```python
from build123d import *

# Parameters (mm, degrees)
BOSS_EXTRUDE1_START     = -3
BOSS_EXTRUDE1_OUTLINE_R = 1.5
BOSS_EXTRUDE1_DEPTH     = 3
FILLET1_R               = 0.5


# Read off the part's stored shape, not the designer's step: Boss-Extrude1
with BuildPart() as part:
    # Boss-Extrude1 outline → Boss-Extrude1 (new body)
    with BuildSketch(Plane.XY.offset(BOSS_EXTRUDE1_START)):
        with BuildLine():
            Line((11.834428484, -2.472731782), (31.256409707, 0.084220555))
            ThreePointArc((31.256409707, 0.084220555), (34.700084383, 4.572104769), (30.212200169, 8.015779445))
            Line((30.212200169, 8.015779445), (13.428337838, 5.806142051))
            ThreePointArc((13.428337838, 5.806142051), (13.411032377, 5.846003182), (13.39360859, 5.885812734))
            ThreePointArc((13.39360859, 5.885812734), (12.04167814, 5.897146383), (10.729304164, 5.572309592))
            Line((10.729304164, 5.572309592), (10.189200244, 6.507557022))
            ThreePointArc((10.189200244, 6.507557022), (11.126720661, 7.481723913), (11.792869471, 8.658240563))
            ThreePointArc((11.792869471, 8.658240563), (11.606759368, 8.906179706), (11.415437385, 9.150119633))
            ThreePointArc((11.415437385, 9.150119633), (10.106597569, 8.81117421), (8.922976471, 8.15773197))
            ThreePointArc((8.922976471, 8.15773197), (8.549706323, 8.548135574), (8.159371308, 8.921477448))
            ThreePointArc((8.159371308, 8.921477448), (8.812813548, 10.105098546), (9.151758972, 11.413938362))
            Line((9.151758972, 11.413938362), (8.659879901, 11.791370448))
            ThreePointArc((8.659879901, 11.791370448), (7.483516811, 11.125336137), (6.509436976, 10.187999326))
            ThreePointArc((6.509436976, 10.187999326), (6.047829045, 10.468613272), (5.574146563, 10.728326528))
            ThreePointArc((5.574146563, 10.728326528), (5.898805358, 12.040487702), (5.887415057, 13.392168338))
            Line((5.887415057, 13.392168338), (5.314609747, 13.629432066))
            ThreePointArc((5.314609747, 13.629432066), (4.351003751, 12.681995862), (3.65280527, 11.524977816))
            ThreePointArc((3.65280527, 11.524977816), (3.134170467, 11.676689406), (2.609274564, 11.805074597))
            ThreePointArc((2.609274564, 11.805074597), (2.58305967, 13.15599481), (2.222297371, 14.458117388))
            Line((2.222297371, 14.458117388), (1.607601557, 14.539043627))
            ThreePointArc((1.607601557, 14.539043627), (0.922327421, 13.375148622), (0.547316802, 12.077605074))
            ThreePointArc((0.547316802, 12.077605074), (0.006856042, 12.089998056), (-0.533618427, 12.078218055))
            ThreePointArc((-0.533618427, 12.078218055), (-0.908651119, 13.375486662), (-1.593822374, 14.539142845))
            Line((-1.593822374, 14.539142845), (-2.208518188, 14.458216606))
            ThreePointArc((-2.208518188, 14.458216606), (-2.569071942, 13.157522433), (-2.595800172, 11.808044777))
            ThreePointArc((-2.595800172, 11.808044777), (-3.121351418, 11.680122659), (-3.640655008, 11.528821757))
            ThreePointArc((-3.640655008, 11.528821757), (-4.338480819, 12.683812024), (-5.300881923, 13.629722958))
            Line((-5.300881923, 13.629722958), (-5.873687233, 13.39245923))
            ThreePointArc((-5.873687233, 13.39245923), (-5.885433032, 12.043808909), (-5.562611018, 10.734312212))
            ThreePointArc((-5.562611018, 10.734312212), (-6.037455135, 10.474599539), (-6.500199913, 10.193895285))
            ThreePointArc((-6.500199913, 10.193895285), (-7.47268922, 11.127885908), (-8.646251294, 11.791833189))
            Line((-8.646251294, 11.791833189), (-9.138130365, 11.414401103))
            ThreePointArc((-9.138130365, 11.414401103), (-8.80083054, 10.109699304), (-8.150983569, 8.92914144))
            ThreePointArc((-8.150983569, 8.92914144), (-8.542690029, 8.555147402), (-8.917254459, 8.163986338))
            ThreePointArc((-8.917254459, 8.163986338), (-10.097571821, 8.813551755), (-11.401949093, 9.15072269))
            Line((-11.401949093, 9.15072269), (-11.779381179, 8.658843619))
            ThreePointArc((-11.779381179, 8.658843619), (-11.116550367, 7.486781519), (-10.184349411, 6.515145975))
            ThreePointArc((-10.184349411, 6.515145975), (-10.46607819, 6.052215075), (-10.726778871, 5.577124264))
            ThreePointArc((-10.726778871, 5.577124264), (-12.034053776, 5.89841947), (-13.38017907, 5.886378776))
            Line((-13.38017907, 5.886378776), (-13.617442798, 5.313573465))
            ThreePointArc((-13.617442798, 5.313573465), (-12.674640857, 4.353631081), (-11.523783462, 3.656571444))
            ThreePointArc((-11.523783462, 3.656571444), (-11.67614775, 3.13618777), (-11.805025713, 2.60949572))
            ThreePointArc((-11.805025713, 2.60949572), (-13.149945407, 2.581153618), (-14.44612812, 2.221261089))
            Line((-14.44612812, 2.221261089), (-14.527054359, 1.606565275))
            ThreePointArc((-14.527054359, 1.606565275), (-13.368714152, 0.923687604), (-12.07756623, 0.548173302))
            ThreePointArc((-12.07756623, 0.548173302), (-12.089998597, 0.005825389), (-12.07808888, -0.536534252))
            ThreePointArc((-12.07808888, -0.536534252), (-13.369010177, -0.912066026), (-14.527153576, -1.594858655))
            Line((-14.527153576, -1.594858655), (-14.446227337, -2.20955447))
            ThreePointArc((-14.446227337, -2.20955447), (-13.151251636, -2.569269431), (-11.807551859, -2.598041398))
            ThreePointArc((-11.807551859, -2.598041398), (0.064079741, -12.08983018), (11.834428484, -2.472731782))
        make_face()
        Circle(BOSS_EXTRUDE1_OUTLINE_R, mode=Mode.SUBTRACT)
        with Locations((30.734304938, 4.05)):
            Circle(BOSS_EXTRUDE1_OUTLINE_R, mode=Mode.SUBTRACT)
    extrude(amount=BOSS_EXTRUDE1_DEPTH)

    # Fillet1
    fillet1_edges = [part.edges().sort_by_distance(p)[0] for p in [
        (29.234304938, 4.05, -3),
        (29.234304938, 4.05, 0),
        (-1.5, 0, 0),
        (-1.5, 0, -3),
    ]]
    fillet(fillet1_edges, radius=FILLET1_R)


solid = part.part
```
Check sheet for the modelled part. Datum: model origin and axes. Units: mm. A direction names the side the tool comes from. Coordinates: 2 decimals unless noted, no trailing zeros. Write each loop counter-clockwise with the first axis right and the second up, starting at its lowest first coordinate (ties: lowest second). Pieces come first, ordered by that corner, then holes. Notation, with made-up numbers: (-10, 40.5) - (38, 40.5) arc R22 ccw to (38, 48.5) - close; hole circle Ø4 at (65.25, 68). An arc over 180 degrees is marked (long way). One line per question, with ' | ' between items.
Item 1: Sectioned sample at C-C on x = 24.5. Record the boundary of the cut face in (y, z).
Determined:
outline: (-0.81, -3) - (7.26, -3) - (7.26, 0) - (-0.81, 0) - close
Item 2: Mould release check, pull along X, two halves, no side actions. Record for faces 6 (the face through (21.409, -1.212, -1.521)), 7 (the face through (-10.08, 8.807, -1.521)), 8 (the face through (-13.386, 0.931, -1.521)): pulls with the +X half, pulls with the -X half, needs draft (parallel to the pull), parting line crosses it, or undercut.
Determined:
face 6: pulls with the +X half | face 7: undercut | face 8: pulls with the -X half
Item 3: Access from +Z, -Z, +X, -X, +Y, -Y to the whole of each face (thin tool, end or side, straight path). Record for faces 1 (the face through (-11.128, 7.502, -1.521)), 2 (the face through (4, 1, -3)), 3 (the face through (4, 1, 0)), 4 (the face through (10.463, 6.033, -1.521)), 5 (the face through (-0.9, 13.36, -1.52)).
Determined:
face 1: +Z, -Z, -X | face 2: -Z, +X, -X, +Y, -Y | face 3: +Z, +X, -X, +Y, -Y | face 4: +Z, -Z | face 5: +Z, -Z, +Y
Item 4: Thickness scan on line 1 (Y direction, x = 0, z = -1.95); line 2 (X direction, y = -4, z = -2.8); line 3 (Y direction, x = -12, z = -2). Record the ranges inside material, lowest first. Write a range as [from, to].
Determined:
line 1: y = [-12.09, -1.5], [1.5, 12.09] | line 2: x = [-11.41, 11.41] | line 3: y = [-2.61, 2.63], [3.9, 5.89]
Item 5: Sectioned sample at D-D on y = -8.25. Record the boundary of the cut face in (x, z), plus the area to 3 significant figures.
Determined:
outline: (-8.84, -3) - (8.84, -3) - (8.84, 0) - (-8.84, 0) - close | area: 53.0 mm2
Item 6: Gauge pin test, flat end, axial feed: P1, Ø3.5, axis at x = 30.73, y = 4.05, coming from the +Z side. Record the tip position at first contact, or that the pin passes through.
Determined:
P1: stops at z = -0.06
Item 7: Sectioned sample at A-A on x = 0. Record the boundary of the cut face in (y, z).
Determined:
outline: (-12.09, -3) - (-2, -3) arc R0.5 ccw to (-1.5, -2.5) - (-1.5, -0.5) arc R0.5 ccw to (-2, 0) - (-12.09, 0) - close; (1.5, -2.5) arc R0.5 ccw to (2, -3) - (12.09, -3) - (12.09, 0) - (2, 0) arc R0.5 ccw to (1.5, -0.5) - close
Item 8: Sectioned sample at B-B on z = -1.55. Give the number of separate pieces and of enclosed holes in the cut face, plus the area to 3 significant figures.
Determined:
separate pieces: 1 | enclosed holes: 2 | area: 668 mm2
